Autodesk Inventor part; units mm, degrees
ref_plane "YZ Plane" through (0, 0, 0) normal (1, 0, 0) x (0, 1, 0)
ref_plane "XZ Plane" through (0, 0, 0) normal (0, 1, 0) x (-1, 0, 0)
ref_plane "XY Plane" through (0, 0, 0) normal (0, 0, 1) x (1, 0, 0)
sketch "Szkic1" plane through (0, 0, 0) normal (1, 0, 0) x (0, 1, 0)
  circle A0 centre (0, 0) radius 16.5
  arc A1 (16.0869, 63.5) -> (15.2371, 62.2084) centre (20, 60) ccw construction
  arc A2 (-20.25, 65.244) -> (-15.2371, 62.2084) centre (-20, 60) ccw
  line L0 (20.25, 69.5) -> (-20.25, 69.5)
  line L1 (-20.25, 69.5) -> (-20.25, 65.244)
  line L2 (-20.25, 63.5) -> (-16.0869, 63.5) construction
  line L3 (20.25, 63.5) -> (20.25, 65.244) construction
  line L4 (16.0869, 63.5) -> (20.25, 63.5) construction
  line L5 (20.25, 65.244) -> (20.25, 69.5)
  line L6 (-20.25, 65.244) -> (-20.25, 63.5) construction
  line L7 (-16.0869, 63.5) -> (-13, 63.5) construction
  arc A3 (20.25, 65.244) -> (16.0869, 63.5) centre (20, 60) ccw construction
  arc A4 (-16.0869, 63.5) -> (-20.25, 65.244) centre (-20, 60) ccw construction
  line L8 (-15.2371, 62.2084) -> (-13, 63.5)
  line L9 (13, 63.5) -> (15.2371, 62.2084)
  arc A5 (15.2371, 62.2084) -> (20.25, 65.244) centre (20, 60) ccw
  line L10 (13, 63.5) -> (16.0869, 63.5) construction
  arc A6 (-15.2371, 62.2084) -> (-16.0869, 63.5) centre (-20, 60) ccw construction
  line L11 (-13, 63.5) -> (13, 63.5)
  line L12 (16.5, 0) -> (-16.5, 0) construction
  arc A7 (15.2371, -62.2084) -> (16.0869, -63.5) centre (20, -60) ccw construction
  arc A8 (-15.2371, -62.2084) -> (-20.25, -65.244) centre (-20, -60) ccw
  line L13 (20.25, -69.5) -> (-20.25, -69.5)
  line L14 (-20.25, -69.5) -> (-20.25, -65.244)
  line L15 (-20.25, -63.5) -> (-16.0869, -63.5) construction
  line L16 (20.25, -63.5) -> (20.25, -65.244) construction
  line L17 (16.0869, -63.5) -> (20.25, -63.5) construction
  line L18 (20.25, -65.244) -> (20.25, -69.5)
  line L19 (-20.25, -65.244) -> (-20.25, -63.5) construction
  line L20 (-16.0869, -63.5) -> (-13, -63.5) construction
  arc A9 (16.0869, -63.5) -> (20.25, -65.244) centre (20, -60) ccw construction
  arc A10 (-20.25, -65.244) -> (-16.0869, -63.5) centre (-20, -60) ccw construction
  line L21 (-15.2371, -62.2084) -> (-13, -63.5)
  line L22 (13, -63.5) -> (15.2371, -62.2084)
  arc A11 (20.25, -65.244) -> (15.2371, -62.2084) centre (20, -60) ccw
  line L23 (13, -63.5) -> (16.0869, -63.5) construction
  arc A12 (-16.0869, -63.5) -> (-15.2371, -62.2084) centre (-20, -60) ccw construction
  line L24 (-13, -63.5) -> (13, -63.5)
  line L25 (24.5, 75.5) -> (-19, 75.5)
  line L26 (-40, 75.5) -> (-40, -75.5)
  line L27 (-19, -75.5) -> (24.5, -75.5)
  line L28 (30.5, -69.5) -> (30.5, -31.5)
  arc A13 (30.5, 69.5) -> (24.5, 75.5) centre (24.5, 69.5) ccw
  arc A14 (24.5, -75.5) -> (30.5, -69.5) centre (24.5, -69.5) ccw
  line L29 (-40, 75.5) -> (-25, 75.5) construction
  line L30 (-25, 81.5) -> (-25, 94.5)
  line L31 (-31, 100.5) -> (-40, 100.5)
  line L32 (-40, 100.5) -> (-40, 75.5)
  arc A15 (-25, 94.5) -> (-31, 100.5) centre (-31, 94.5) ccw
  arc A16 (-25, 81.5) -> (-19, 75.5) centre (-19, 81.5) ccw
  line L33 (-40, -75.5) -> (-25, -75.5) construction
  line L34 (-25, -81.5) -> (-25, -94.5)
  line L35 (-31, -100.5) -> (-40, -100.5)
  line L36 (-40, -100.5) -> (-40, -75.5)
  arc A17 (-31, -100.5) -> (-25, -94.5) centre (-31, -94.5) ccw
  arc A18 (-19, -75.5) -> (-25, -81.5) centre (-19, -81.5) ccw
  line L37 (30.5, 25.5) -> (30.5, -25.5) construction
  line L38 (30.5, 31.5) -> (30.5, 69.5)
  line L39 (30.5, -31.5) -> (30.5, 31.5)
  circle A19 centre (0, 0) radius 18.5
  point P0 (-25, 100.5)
  point P1 (-25, -100.5)
  dimension "d0" = 33
  dimension "d1" = 10.5
  dimension "d3" = 20
  dimension "d4" = 60
  dimension "d6" = 6
  dimension "d8" = 3.5
  dimension "d9" = 150
  dimension "d10" = 150
  dimension "d11" = 26
  dimension "d12" = 13
  dimension "d13" = 6
  dimension "d14" = 6
  dimension "d15" = 10.5
  dimension "d16" = 20
  dimension "d17" = 6
  dimension "d18" = 15
  dimension "d19" = 25
  dimension "d20" = 6
  dimension "d21" = 15
  dimension "d22" = 25
  dimension "d23" = 6
  dimension "d50" = 37
  dimension "d55" = 40
  dimension "d56" = 0.25
  dimension "d57" = 0.25
extrude "Wyciągnięcie proste1" add sketch "Szkic1" along normal blind 45 contours A0 | L1 L0 L5 A5 L9 L11 L8 A2 | L21 L24 L22 A11 L18 L13 L14 A8 | A13 L38 L39 L28 A14 L27 A18 L34 A17 L35 L36 L26 L32 L31 A15 L30 A16 L25 | A19
extrude "Wyciągnięcie proste4" cut sketch "Szkic1" along normal through all contours A0 | L1 L0 L5 A5 L9 L11 L8 A2 | L21 L24 L22 A11 L18 L13 L14 A8
extrude "Wyciągnięcie proste7" cut sketch "Szkic1" along normal blind 7 contours A19
sketch "Szkic2" plane through (0, -25, 94.5) normal (0, 1, 0) x (1, 0, 0)
  circle A0 centre (37, 6.5) radius 5.5
  circle A1 centre (8, 6.5) radius 5.5
  circle A2 centre (37, 6.5) radius 3.25
  circle A3 centre (8, 6.5) radius 3.25
  line L0 (45, 13) -> (45, 0)
  line L1 (0, -6) -> (45, -6)
  line L2 (0, 13) -> (0, 0)
  point P0 (0, 94.5)
  dimension "d41" = 6.5
  dimension "d42" = 11
  dimension "d43" = 8
  dimension "d44" = 12.5
  dimension "d45" = 8
extrude "Wyciągnięcie proste5" cut sketch "Szkic2" against normal through all contours A2 | A3
extrude "Wyciągnięcie proste6" cut sketch "Szkic2" against normal blind 5
sketch "Szkic3" plane through (0, -19, 75.5) normal (0, 0, 1) x (1, 0, 0)
  line L0 (45, 32) -> (45, 6)
  line L1 (0, 32) -> (45, 32)
  line L2 (0, 6) -> (0, 32)
  line L3 (0, 6) -> (45, 6)
  line L4 (0, 6) -> (45, 6)
  line L5 (0, 32) -> (45, 6) construction
  line L6 (45, 32) -> (0, 6) construction
  circle A0 centre (22.5, 19) radius 3.25
  circle A1 centre (22.5, 19) radius 5.5
  point P0 (0, 19)
  dimension "d58" = 6.5
  dimension "d59" = 11
extrude "Wyciągnięcie proste9" cut sketch "Szkic3" against normal blind 60 contours A0
sketch "Szkic4" plane through (45, 0, 0) normal (1, 0, 0) x (0, 0, -1)
  line L0 (-35.5, 5.25) -> (-30, 5.25)
  line L1 (-30, 5.25) -> (-30, -5.25)
  line L2 (-30, -5.25) -> (-35.5, -5.25)
  line L3 (-35.5, -5.25) -> (-35.5, 5.25)
  line L4 (-75.5, 24.5) -> (-75.5, -19)
  point P0 (0, 0)
  dimension "d62" = 10.5
  dimension "d63" = 5.25
  dimension "d64" = 40
  dimension "d65" = 5.5
extrude "Wyciągnięcie proste10" cut sketch "Szkic4" against normal blind 28.75
mirror "Odbij3" about plane through (0, 0, 0) normal (0, 0, 1) of "Wyciągnięcie proste10", "Wyciągnięcie proste9", "Wyciągnięcie proste6", "Wyciągnięcie proste5"
equation "\"d14\" = d13"
properties part number "Y_motor_mount"
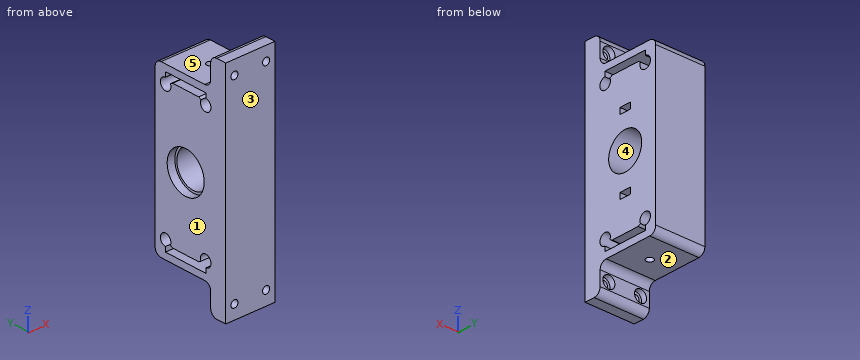
Check sheet for the modelled part. Datum: model origin and axes. Units: mm. Face numbers are marked on the shaded views. A direction names the side the tool comes from. Give positions to 0.01 mm unless a question says otherwise; leave off trailing zeros. Write each loop counter-clockwise with the first axis right and the second up, starting at its lowest first coordinate (ties: lowest second). Pieces come first, ordered by that corner, then holes. Notation, with made-up numbers: (4, -32) - (55, -32) arc R28 ccw to (55, -6) - close; hole circle Ø11 at (60.25, -31.5). An arc over 180 degrees is marked (long way). Answer as a JSON object with one key per item and string values. Group by question number.
1) Depth check by flat-ended pin: P1, Ø11.5, axis at x = 31.5, y = -2.5, coming from the +Z side; P2, Ø10, axis at x = 39, y = 7.5, coming from the -Z side; P3, Ø6, axis at x = 22.5, y = 0, coming from the -Z side; P4, Ø14.5, axis at x = 13, z = -90.5, coming from the +Y side. Enter the tip coordinate at first touch or a pass-through.
2) Thickness scan on probe 1 along X at (y, z) = (-35.5, -88); probe 2 along Z at (x, y) = (5, 0); probe 3 along Z at (x, y) = (18.5, 0). Record the ranges inside material, lowest first. Write a range as from..to.
3) Sectioned sample at D-D (x = 37). Give the number of separate pieces and of enclosed holes in the cut face, then the cut area to 3 significant figures.
4) Access from +Z, -Z, +X, -X, +Y, -Y to the whole of each face (thin tool, end or side, straight path). Record for the marked faces 1 and 2.
5) Release check for a two-part mould opening along Z. For the marked faces 3, 4 and 5 record: pulls with the +Z half, pulls with the -Z half, needs draft (parallel to the pull), parting line crosses it, or undercut.
6) Sectioned sample at A-A (z = 0). Record the cut outline in (x, y).
7) Sectioned sample at B-B (z = 88). Record the cut outline in (x, y).
8) Sectioned sample at C-C (y = -9). Record the cut outline in (x, z), then the cut area to 3 significant figures.
Geometry results:
{
 "1": {"P1": "stops at z = 75.5", "P2": "stops at z = -75.5", "P3": "passes through", "P4": "stops at y = -25"},
 "2": {"probe 1": "x = 0..4.75, 11.25..33.75, 40.25..45", "probe 2": "z = -75.5..-69.5, -63.5..-18.5, 18.5..63.5, 69.5..75.5", "probe 3": "z = -75.5..-69.5, -63.5..-35.5, -30..-16.5, 16.5..30, 35.5..63.5, 69.5..75.5"},
 "3": {"separate pieces": "3", "enclosed holes": "5", "area": "9,350 mm^2"},
 "4": {"face 1": "+Z, -Z, -X, +Y, -Y", "face 2": "-Z, +X, -X, +Y"},
 "5": {"face 3": "needs draft", "face 4": "undercut", "face 5": "pulls with the +Z half"},
 "6": {"outline": "(0, -40) - (45, -40) - (45, -16.5) - (7, -16.5) - (7, -18.5) - (0, -18.5) - close; (0, 18.5) - (7, 18.5) - (7, 16.5) - (45, 16.5) - (45, 30.5) - (0, 30.5) - close"},
 "7": {"outline": "(0, -40) - (4.75, -40) - (4.75, -30) - (2.5, -30) - (2.5, -25) - (0, -25) - close; (11.25, -40) - (33.75, -40) - (33.75, -30) - (31.5, -30) - (31.5, -25) - (13.5, -25) - (13.5, -30) - (11.25, -30) - close; (40.25, -40) - (45, -40) - (45, -25) - (42.5, -25) - (42.5, -30) - (40.25, -30) - close"},
 "8": {"outline": "(0, -75.5) - (45, -75.5) - (45, -69.5) - (0, -69.5) - close; (0, -63.5) - (45, -63.5) - (45, -13.83) - (7, -13.83) - (7, -16.16) - (0, -16.16) - close; (0, 16.16) - (7, 16.16) - (7, 13.83) - (45, 13.83) - (45, 63.5) - (0, 63.5) - close; (0, 69.5) - (45, 69.5) - (45, 75.5) - (0, 75.5) - close", "area": "4,980 mm^2"}
}
